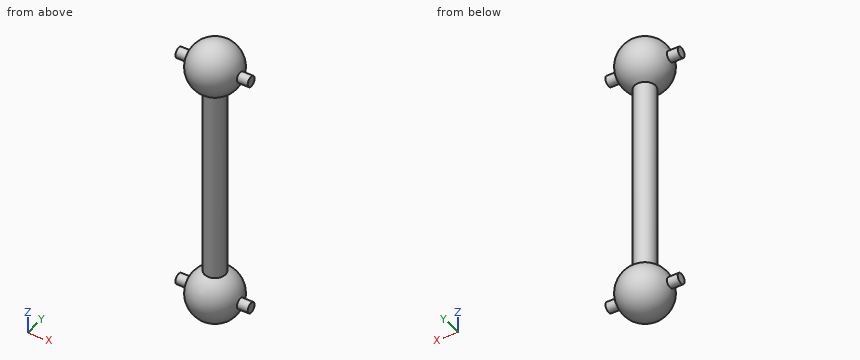
```python
from build123d import *

# Parameters (mm, degrees)
F1_R          = 1
F2_DEPTH      = 23
F7_R          = 0.5
F8_DEPTH      = 3.5
F8_DEPTH_BACK = 3.5


with BuildPart() as f2:
    # F1 (on Top) → F2 (new body)
    with BuildSketch(Plane.XY):
        Circle(F1_R)
    extrude(amount=F2_DEPTH)

    # F3 (on Right) → F4 (revolve)
    with BuildSketch(Plane.YZ):
        with BuildLine():
            Line((-0.5, 0), (-0.5, 2.4494897428))
            ThreePointArc((-0.5, 2.4494897428), (-2.4873403825, -0.251272405), (0, -2.5))
            Line((0, -2.5), (0, 0))
            Line((0, 0), (-0.5, 0))
        make_face()
    revolve(axis=Axis((0, 0, -1.25), (0, 0, 1)))

    # F5 (on Front) → F6 (revolve)
    with BuildSketch(Plane.XZ):
        with BuildLine():
            Line((0, 23), (0, 25.5))
            ThreePointArc((0, 25.5), (-2.4472657823, 23.5107741092), (-1, 20.7087121525))
            Line((-1, 20.7087121525), (-1, 23))
            Line((-1, 23), (0, 23))
        make_face()
    revolve(axis=Axis((0, 0, 24.25), (0, 0, 1)))

    # F7 (on Right) → F8 (join, two sides)
    with BuildSketch(Plane.YZ) as f8_sk:
        Circle(F7_R)
        with Locations((0, 23)):
            Circle(F7_R)
    extrude(amount=F8_DEPTH)
    extrude(f8_sk.sketch, amount=-F8_DEPTH_BACK)


solid = f2.part
```
Build history of the part. All positions in model axes, mm. Round coordinates to 2 decimals unless told otherwise and drop trailing zeros. Order: outer loops, then holes, each group sorted by start corner. A loop starts at its lowest first (then second) coordinate and runs counter-clockwise, first axis right, second up. Notation, with made-up numbers: (63.5, -37) -> (110.5, -37) arc R16 ccw to (110.5, -12) -> close; hole circle Ø8 at (-22.5, 28). An arc over 180 degrees is marked (long way). Answer in a Markdown table with one row per item.
1) Wall check: L1, parallel to X at y = -0.1, z = 7.5; L2, parallel to Z at x = -1.5, y = 0.95; L3, parallel to Z at x = 1, y = -1.85. Give the ranges that are in metal, low to high.
Values:
| item | result |
|---|---|
| L1 | -0.99 to 0.99 |
| L2 | -1.76 to 1.76, 21.24 to 24.76 |
| L3 | -1.35 to 1.35, 21.65 to 24.35 |
2) Band-saw the part on B-B on x = 2.75. Give the cut face in (y, z), and give its area (3 significant figures).
Values:
| item | result |
|---|---|
| outline | circle Ø1 at (0, 0); circle Ø1 at (0, 23) |
| area | 1.57 mm2 |
3) Pin check, flat tips, straight feed: P1, Ø4, axis at x = -2.5, z = 19, coming from the +Y side; P2, Ø3, axis at y = 1.5, z = 20.5, coming from the +X side; P3, Ø3, axis at x = 3, y = 2, coming from the -Z side; P4, Ø1, axis at x = 2, z = 3, coming from the -Y side. Stop position of each tip, or through.
Values:
| item | result |
|---|---|
| P1 | y = 0.87 |
| P2 | x = 2.06 |
| P3 | z = -1.35 |
| P4 | through |
4) Band-saw the part on C-C on z = 23. Give the cut face in (x, y).
Values:
| item | result |
|---|---|
| outline | (-3.5, -0.5) -> (-2.45, -0.5) arc R2.5 ccw to (2.45, -0.5) -> (3.5, -0.5) -> (3.5, 0.5) -> (2.45, 0.5) arc R2.5 ccw to (-2.45, 0.5) -> (-3.5, 0.5) -> close |
5) Band-saw the part on A-A on y = 0. Give the cut face in (x, z), and give its area (3 significant figures).
Values:
| item | result |
|---|---|
| outline | (-3.5, -0.5) -> (-2.45, -0.5) arc R2.5 ccw to (2.45, -0.5) -> (3.5, -0.5) -> (3.5, 0.5) -> (2.45, 0.5) arc R2.5 ccw to (1, 2.29) -> (1, 20.71) arc R2.5 ccw to (2.45, 22.5) -> (3.5, 22.5) -> (3.5, 23.5) -> (2.45, 23.5) arc R2.5 ccw to (-2.45, 23.5) -> (-3.5, 23.5) -> (-3.5, 22.5) -> (-2.45, 22.5) arc R2.5 ccw to (-1, 20.71) -> (-1, 2.29) arc R2.5 ccw to (-2.45, 0.5) -> (-3.5, 0.5) -> close |
| area | 79.6 mm2 |
6) Band-saw the part on D-D on y = 1.45. Give the cut face in (x, z).
Values:
| item | result |
|---|---|
| outline | circle Ø4.07 at (0, 0); circle Ø4.07 at (0, 23) |
